from build123d import *

# Parameters (mm, degrees)
SKETCH_1_W          = 25.58
SKETCH_1_H          = 20
EXTRUDE_1_DEPTH     = 15
SKETCH_4_W          = 25.58
SKETCH_4_H          = 15
CUT_EXTRUDE_3_DEPTH = 7
SKETCH_5_W          = 5
SKETCH_5_H          = 5
CUT_EXTRUDE_4_DEPTH = 32.294350928
CUT_EXTRUDE_5_REACH = 30.082
SKETCH_6_W          = 5
SKETCH_6_H          = 5
HOLE_WIZARD_M2_1_D  = 2.4
SKETCH_10_W         = 17
SKETCH_10_H         = 12
CUT_EXTRUDE_7_DEPTH = 25.770629786


with BuildPart() as part:
    # ｽｹｯﾁ1 → ﾎﾞｽ - 押し出し1 (new body)
    with BuildSketch(Plane.XY):
        Rectangle(SKETCH_1_W, SKETCH_1_H)
    extrude(amount=EXTRUDE_1_DEPTH)

    # ｽｹｯﾁ4 → ｶｯﾄ - 押し出し3 (cut)
    with BuildSketch(Plane.XY.offset(15)):
        with Locations((0, 2.5)):
            Rectangle(SKETCH_4_W, SKETCH_4_H)
    extrude(amount=-CUT_EXTRUDE_3_DEPTH, mode=Mode.SUBTRACT)

    # ｽｹｯﾁ5 → ｶｯﾄ - 押し出し4 (cut, through all)
    with BuildSketch(Plane(origin=(12.79, 0, 0), x_dir=(0, 0, -1), z_dir=(1, 0, 0))):
        with Locations((-5.5, -2.5)):
            Rectangle(SKETCH_5_W, SKETCH_5_H)
    extrude(amount=-CUT_EXTRUDE_4_DEPTH, mode=Mode.SUBTRACT)

    # ｽｹｯﾁ6 → ｶｯﾄ - 押し出し5 (cut, up to next)
    with BuildSketch(Plane(origin=(0, 10, 0), x_dir=(1, 0, 0), z_dir=(0, 1, 0)), mode=Mode.PRIVATE) as cut_extrude_5_sk1:
        with Locations((0, -5.5)):
            Rectangle(SKETCH_6_W, SKETCH_6_H)
    cut_extrude_5_tool1 = extrude(cut_extrude_5_sk1.sketch, amount=-CUT_EXTRUDE_5_REACH, mode=Mode.PRIVATE) & part.part
    add(cut_extrude_5_tool1.solids().sort_by_distance((0, 10, 5.5))[0], mode=Mode.SUBTRACT)

    # M2 すきま穴1 (through all)
    with Locations(Plane(origin=(0, -5, 0), x_dir=(1, 0, 0), z_dir=(0, 1, 0))):
        with Locations((10.5, -12), (-10.5, -12)):
            Hole(HOLE_WIZARD_M2_1_D / 2)

    # ｽｹｯﾁ10 → ｶｯﾄ - 押し出し7 (cut, through all)
    with BuildSketch(Plane(origin=(0, -5, 0), x_dir=(1, 0, 0), z_dir=(0, 1, 0))):
        with Locations((0, -9)):
            Rectangle(SKETCH_10_W, SKETCH_10_H)
    extrude(amount=-CUT_EXTRUDE_7_DEPTH, mode=Mode.SUBTRACT)


solid = part.part
Geometry check sheet. Reference: the model listing, model coordinates, mm. A direction names the side the tool comes from. Coordinates: 2 decimals unless noted, no trailing zeros. Order: outer loops, then holes, each group sorted by start corner. A loop starts at its lowest first (then second) coordinate and runs counter-clockwise, first axis right, second up. Notation, with made-up numbers: (82.25, 33) - (114.25, 33) arc R15 ccw to (114.25, 39) - close; hole circle Ø1 at (83, 51). An arc over 180 degrees is marked (long way). Answer in a Markdown table with one row per item. Add a question column.
1) Material ranges on line 1 along X through (y, z) = (-8.65, 12); line 2 along Y through (x, z) = (9, 5); line 3 along X through (y, z) = (7.25, 5), recorded low to high. Write a range as [from, to].
2) Cross-section at A-A, the plane z = 5.75. Record the cut outline in (x, y).
3) Cross-section at D-D, the plane y = -6.25. Record the cut outline in (x, z), then the cut area to 3 significant figures.
4) Gauge pin test, flat ends, axial feed: P1, Ø4, axis at x = 10.5, z = 12, coming from the +Y side; P2, Ø8, axis at x = -3.5, z = 12.5, coming from the -Y side; P3, Ø3, axis at x = 9, y = 6, coming from the +Z side. Record the tip position at first contact, or that the pin passes through.
5) Set-up check for faces 4 (the flat face through (-8, 0, 6)), 5 (the flat face through (8, 5, 8)), 6 (the flat face through (2.5, 5, 6)), 7 (the flat face through (-8.5, -7, 9)): record each of +Z, -Z, +X, -X, +Y, -Y from which the full face is reachable in a straight line by a thin tool's end or side.
6) Release check for a two-part mould opening along Y. For faces 1 (the flat face through (0, 10, 2)), 2 (the flat face through (0, -2, 3)), 3 (the flat face through (11, -7, 15)) record: +Y half, -Y half, draft (parallel to the pull), parting line (faces both ways), or undercut.
7) Cross-section at B-B, the plane x = 10.5. Record the cut outline in (y, z).
8) Cross-section at C-C, the plane z = 9. Record the cut outline in (x, y).
Check result:
| question | item | result |
|---|---|---|
| 1 | line 1 | x = [-12.79, -11.7], [-9.3, -8.5], [8.5, 9.3], [11.7, 12.79] |
| 1 | line 2 | y = [-10, -5], [0, 10] |
| 1 | line 3 | x = [-12.79, -2.5], [2.5, 12.79] |
| 2 | outline | (-12.79, -10) - (-8.5, -10) - (-8.5, -5) - (-12.79, -5) - close; (-12.79, 0) - (-2.5, 0) - (-2.5, 10) - (-12.79, 10) - close; (2.5, 0) - (12.79, 0) - (12.79, 10) - (2.5, 10) - close; (8.5, -10) - (12.79, -10) - (12.79, -5) - (8.5, -5) - close |
| 3 | outline | (-12.79, 0) - (12.79, 0) - (12.79, 15) - (8.5, 15) - (8.5, 3) - (-8.5, 3) - (-8.5, 15) - (-12.79, 15) - close; hole circle Ø2.4 at (-10.5, 12); hole circle Ø2.4 at (10.5, 12) |
| 3 | area | 171 mm² |
| 4 | P1 | stops at y = -5 |
| 4 | P2 | passes through |
| 4 | P3 | stops at z = 8 |
| 5 | face 4 | +Z, +X, -X |
| 5 | face 5 | +Z, +X, -X, +Y |
| 5 | face 6 | +Z, +Y, -Y |
| 5 | face 7 | +Z, -Y |
| 6 | face 1 | +Y half |
| 6 | face 2 | undercut |
| 6 | face 3 | draft |
| 7 | outline | (-10, 0) - (10, 0) - (10, 8) - (0, 8) - (0, 3) - (-5, 3) - (-5, 10.8) - (-10, 10.8) - close; (-10, 13.2) - (-5, 13.2) - (-5, 15) - (-10, 15) - close |
| 8 | outline | (-12.79, -10) - (-8.5, -10) - (-8.5, -5) - (-12.79, -5) - close; (8.5, -10) - (12.79, -10) - (12.79, -5) - (8.5, -5) - close |
